Check sheet for the modelled part. Datum: model origin and axes. Units: mm. Face numbers are marked on the shaded views. A direction names the side the tool comes from. Round coordinates to 2 decimals unless told otherwise and drop trailing zeros. Order: outer loops, then holes, each group sorted by start corner. A loop starts at its lowest first (then second) coordinate and runs counter-clockwise, first axis right, second up. Notation, with made-up numbers: (14.5, 48) -> (29.5, 48) arc R17 cw to (29.5, 58) -> close; hole circle Ø11 at (53.5, 1.25). An arc over 180 degrees is marked (long way). Answer in a Markdown table with one row per item. Add a question column.
1. Access from +Z, -Z, +X, -X, +Y, -Y to the whole of each face (thin tool, end or side, straight path). Record for the marked faces 1, 2 and 3.
2. Material ranges on L1, parallel to Z at x = -5.5, y = 6.25; L2, parallel to Y at x = -15, z = 11 (3 decimals), recorded low to high. Write a range as from..to.
3. Sectioned sample at C-C, the plane y = 1. Record the boundary of the cut face in (x, z), then the cut area to 3 significant figures.
4. Depth check by flat-ended pin: P1, Ø4, axis at x = -13.5, z = 37, coming from the +Y side (3 decimals); P2, Ø1.6, axis at y = 5, z = -27.5, coming from the +X side; P3, Ø3, axis at x = 6.5, z = -16, coming from the -Y side; P4, Ø2, axis at y = 2.5, z = 47, coming from the +X side. Enter the tip coordinate at first touch or a pass-through.
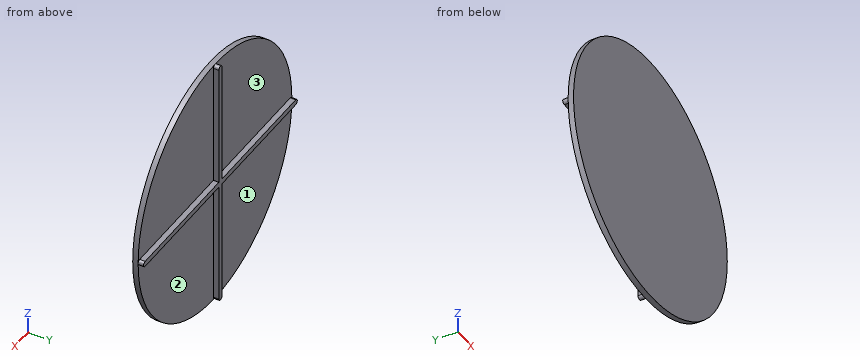
```python
from build123d import *

# Parameters (mm, degrees)
SKETCH1_R           = 76.2
BOSS_EXTRUDE1_DEPTH = 3.175
BOSS_EXTRUDE2_DEPTH = 3.175


with BuildPart() as part:
    # Sketch1 → Boss-Extrude1 (new body)
    with BuildSketch(Plane(origin=(0, 0, 0), x_dir=(1, 0, 0), z_dir=(0, 1, 0))):
        Circle(SKETCH1_R)
    extrude(amount=BOSS_EXTRUDE1_DEPTH)

    # Sketch2 → Boss-Extrude2 (add)
    with BuildSketch(Plane(origin=(0, 3.175, 0), x_dir=(1, 0, 0), z_dir=(0, 1, 0))):
        with BuildLine():
            Line((-74.6125, 1.5875), (74.6125, 1.5875))
            ThreePointArc((74.6125, 1.5875), (76.2, 0), (74.6125, -1.5875))
            Line((74.6125, -1.5875), (-74.6125, -1.5875))
            ThreePointArc((-74.6125, -1.5875), (-76.2, 0), (-74.6125, 1.5875))
        make_face()
        with BuildLine():
            Line((1.5875, 74.6125), (1.5875, -74.6125))
            ThreePointArc((1.5875, -74.6125), (0, -76.2), (-1.5875, -74.6125))
            Line((-1.5875, -74.6125), (-1.5875, 74.6125))
            ThreePointArc((-1.5875, 74.6125), (0, 76.2), (1.5875, 74.6125))
        make_face()
    extrude(amount=BOSS_EXTRUDE2_DEPTH)


solid = part.part
```
Answer key:
| question | item | result |
|---|---|---|
| 1 | face 1 | -Z, -X, +Y |
| 1 | face 2 | -Z, +X, +Y |
| 1 | face 3 | +Z, -X, +Y |
| 2 | L1 | z = -1.59..1.59 |
| 2 | L2 | y = 0..3.175 |
| 3 | outline | circle Ø152.4 at (0, 0) |
| 3 | area | 18,200 mm² |
| 4 | P1 | stops at y = 3.175 |
| 4 | P2 | stops at x = 1.59 |
| 4 | P3 | stops at y = 0 |
| 4 | P4 | stops at x = 60.75 |
